from build123d import *

# Parameters (mm, degrees)
BOSS_EXTRUDE1_DEPTH = 150
CUT_EXTRUDE4_REACH  = 1253.709
SKETCH5_W           = 12.933974596
SKETCH5_H           = 32.032750252
SKETCH7_W           = 25
SKETCH7_H           = 18.64
CUT_EXTRUDE5_DEPTH  = 1252.708964453


with BuildPart() as part:
    # Sketch1 → Boss-Extrude1 (new body)
    with BuildSketch(Plane.XY):
        Polygon((-1242.686178465, 885.422015852), (-1240.286178465, 885.422015852), (-1241.186178465, 883.863170125), (-1236.186178465, 883.863170125), (-1237.086178465, 885.422015852), (-1224.152203869, 885.422015852), (-1225.052203869, 883.863170125), (-1220.052203869, 883.863170125), (-1220.952203869, 885.422015852), (-1217.686178465, 885.422015852), (-1217.686178465, 882.893470027), (-1242.686178465, 882.893470027), align=None)
    extrude(amount=BOSS_EXTRUDE1_DEPTH)

    # Cut-Extrude4: up to this face of the body (flat: up to its plane)
    cut_extrude4_end = Plane(part.part.faces().sort_by_distance((-1230.186178465, 882.893470027, 75))[0])
    # Sketch5 → Cut-Extrude4 (cut, up to the picked face)
    with BuildSketch(Plane(origin=(0, 885.422015852, 0), x_dir=(1, 0, 0), z_dir=(0, 1, 0)), mode=Mode.PRIVATE) as cut_extrude4_sk1:
        with Locations((-1230.619191167, -69.852079699)):
            Rectangle(SKETCH5_W, SKETCH5_H)
    cut_extrude4_tool1 = split(extrude(cut_extrude4_sk1.sketch, amount=-CUT_EXTRUDE4_REACH, mode=Mode.PRIVATE), bisect_by=cut_extrude4_end, keep=Keep.BOTH, mode=Mode.PRIVATE)
    add(cut_extrude4_tool1.solids().sort_by(Axis((-1230.619191, 885.422016, 69.85208), (0, -1, 0)))[0], mode=Mode.SUBTRACT)

    # Sketch7 → Cut-Extrude5 (cut, through all)
    with BuildSketch(Plane(origin=(0, 882.893470027, 0), x_dir=(-1, 0, 0), z_dir=(0, -1, 0))):
        with Locations((1230.186178465, -140.68)):
            Rectangle(SKETCH7_W, SKETCH7_H)
    extrude(amount=-CUT_EXTRUDE5_DEPTH, mode=Mode.SUBTRACT)


solid = part.part
Work out the finished part from the listing and answer in its coordinate system (mm). A direction names the side the tool comes from. Round coordinates to 2 decimals unless told otherwise and drop trailing zeros. Loops run counter-clockwise (first coordinate to the right, second up) from the corner with the lowest first, then second, coordinate; pieces in that order, holes last. Notation, with made-up numbers: (4, 75.25) -> (32, 75.25) arc R16 cw to (32, 105.25) -> close; hole circle Ø1 at (6, 39). An arc over 180 degrees is marked (long way). Use one line per item in the form item = value.
(1) Find section A-A on x = -1228. Give the vertices of the cut face in (y, z).
Answer list:
outline = (882.89, 0) -> (885.42, 0) -> (885.42, 53.84) -> (882.89, 53.84) -> close; (882.89, 85.87) -> (885.42, 85.87) -> (885.42, 131.36) -> (882.89, 131.36) -> close
(2) A tool of negligible diameter and unlimited length cuts with its end or side. For faces 1 (the flat face through (-1230, 884, 131.36)), 2 (the flat face through (-1231, 884, 53.836)), from which of +Z, -Z, +X, -X, +Y, -Y can it reach the whole face along a straight path? Write none if from no direction.
Answer list:
face_1 = +Z, +X, -X, +Y, -Y
face_2 = +Y, -Y
(3) Find section D-D on z = 10.5. Give the vertices of the cut face in (x, y).
Answer list:
outline = (-1242.69, 882.89) -> (-1217.69, 882.89) -> (-1217.69, 885.42) -> (-1220.95, 885.42) -> (-1220.05, 883.86) -> (-1225.05, 883.86) -> (-1224.15, 885.42) -> (-1237.09, 885.42) -> (-1236.19, 883.86) -> (-1241.19, 883.86) -> (-1240.29, 885.42) -> (-1242.69, 885.42) -> close
(4) Find section B-B on z = 61. Give the vertices of the cut face in (x, y), then the cut area to 3 significant figures.
Answer list:
outline = (-1242.69, 882.89) -> (-1237.09, 882.89) -> (-1237.09, 883.86) -> (-1241.19, 883.86) -> (-1240.29, 885.42) -> (-1242.69, 885.42) -> close; (-1224.15, 882.89) -> (-1217.69, 882.89) -> (-1217.69, 885.42) -> (-1220.95, 885.42) -> (-1220.05, 883.86) -> (-1224.15, 883.86) -> close
area = 19.1 mm2
(5) For a pull along X with two mould halves and no side action, classify faces 3 (the flat face through (-1230, 884, 0)), 4 (the flat face through (-1231, 884, 85.868)), 5 (the flat face through (-1223, 883.863, 65)), 6 (the flat face through (-1217.686, 884, 65)) as released by +X, released by -X, zero draft, split by the parting line, or undercut.
Answer list:
face_3 = zero draft
face_4 = undercut
face_5 = undercut
face_6 = released by +X
(6) A flat-ended cylindrical pin translates along its axis: P1, Ø1.5, axis at x = -1222.5, z = 46, coming from the +Y side. Find the tip coordinate at first contact, or state that the pin passes through.
Answer list:
P1 = 883.86
(7) Straight lines are drawn through the part: line 1 (Z direction, x = -1227.75, y = 883.3); line 2 (X direction, y = 884.65, z = 26.5); line 3 (X direction, y = 885.25, z = 45). For each, find the intervals that lie inside material, in ascending order.
Answer list:
line_1 = 0 to 53.84, 85.87 to 131.36
line_2 = -1242.69 to -1240.73, -1236.64 to -1224.6, -1220.51 to -1217.69
line_3 = -1242.69 to -1240.39, -1236.99 to -1224.25, -1220.85 to -1217.69
(8) Find section C-C on y = 884.6. Give the vertices of the cut face in (x, z).
Answer list:
outline = (-1242.69, 0) -> (-1240.76, 0) -> (-1240.76, 131.36) -> (-1242.69, 131.36) -> close; (-1236.61, 0) -> (-1224.63, 0) -> (-1224.63, 53.84) -> (-1236.61, 53.84) -> close; (-1236.61, 85.87) -> (-1224.63, 85.87) -> (-1224.63, 131.36) -> (-1236.61, 131.36) -> close; (-1220.48, 0) -> (-1217.69, 0) -> (-1217.69, 131.36) -> (-1220.48, 131.36) -> close
